Could you check a few things on this drawing? It's one solid part, dimensions in mm from its lowest x, y, z. Coordinates: 2 decimals unless noted, no trailing zeros. Write each loop counter-clockwise with the first axis right and the second up, starting at its lowest first coordinate (ties: lowest second). Pieces come first, ordered by that corner, then holes.
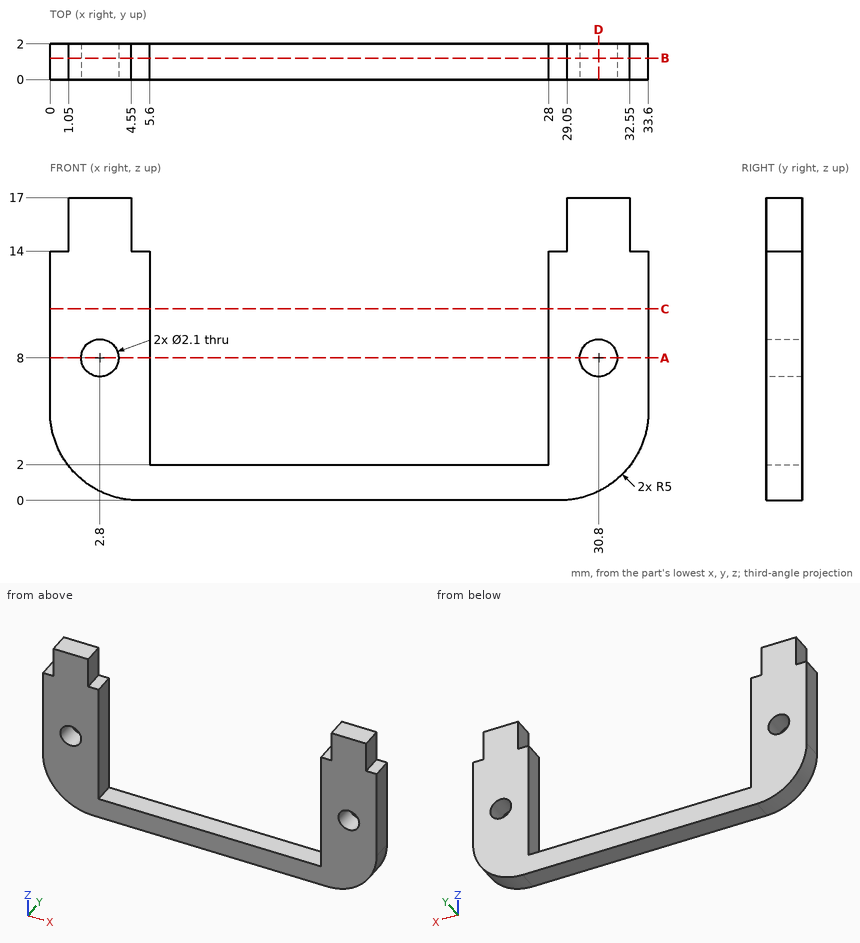
1) I need wall thicknesses on probe 1 along X at (y, z) = (0.65, 8); probe 2 along X at (y, z) = (0.7, 10); probe 3 along Z at (x, y) = (6, 1.7). Which ranges of each line are inside material? Lowest first, please.
Values follow:
probe 1: x = 0 to 1.75, 3.85 to 5.6, 28 to 29.75, 31.85 to 33.6
probe 2: x = 0 to 5.6, 28 to 33.6
probe 3: z = 0 to 2
2) Will these pins go through, and if not, where does the flat tip stop? pin 1 (1 mm diameter, centred on x = 29.5, y = 0.5, fed in from -Z); pin 2 (0.6 mm diameter, centred on y = 1.5, z = 15.5, fed in from -X); pin 3 (0.8 mm diameter, centred on x = 33, y = 0.5, fed in from +Z); pin 4 (3 mm diameter, centred on x = 17.5, z = 4.5, fed in from +Y).
Values follow:
pin 1: stops at z = 0.02
pin 2: stops at x = 1.05
pin 3: stops at z = 14
pin 4: passes through
3) Imagine slicing it at A-A on z = 8. Please give me the cut outline in (x, y), then the cut area to 3 significant figures.
Values follow:
outline: (0, 0) - (1.75, 0) - (1.75, 2) - (0, 2) - close; (3.85, 0) - (5.6, 0) - (5.6, 2) - (3.85, 2) - close; (28, 0) - (29.75, 0) - (29.75, 2) - (28, 2) - close; (31.85, 0) - (33.6, 0) - (33.6, 2) - (31.85, 2) - close
area: 14.0 mm2
4) Imagine slicing it at C-C on z = 10.75. Please give me the cut outline in (x, y).
Values follow:
outline: (0, 0) - (5.6, 0) - (5.6, 2) - (0, 2) - close; (28, 0) - (33.6, 0) - (33.6, 2) - (28, 2) - close
5) Imagine slicing it at D-D on x = 30.8. Please give me the cut outline in (y, z), then the cut area to 3 significant figures.
Values follow:
outline: (0, 0.51) - (2, 0.51) - (2, 6.95) - (0, 6.95) - close; (0, 9.05) - (2, 9.05) - (2, 17) - (0, 17) - close
area: 28.8 mm2
6) Imagine slicing it at B-B on y = 1.2. Please give me the cut outline in (x, z).
Values follow:
outline: (0, 5) arc R5 ccw to (5, 0) - (28.6, 0) arc R5 ccw to (33.6, 5) - (33.6, 14) - (32.55, 14) - (32.55, 17) - (29.05, 17) - (29.05, 14) - (28, 14) - (28, 2) - (5.6, 2) - (5.6, 14) - (4.55, 14) - (4.55, 17) - (1.05, 17) - (1.05, 14) - (0, 14) - close; hole circle Ø2.1 at (2.8, 8); hole circle Ø2.1 at (30.8, 8)
